```python
from build123d import *

# Parameters (mm, degrees)
EXTRUDE032_DEPTH           = 3
EXTRUDE033_DEPTH           = 3
CYLINDER057_R              = 4
CYLINDER057_DEPTH          = 12
CYLINDER055_R              = 4
CYLINDER055_DEPTH          = 12
CYLINDER053_R              = 1.85
CYLINDER053_DEPTH          = 12
CYLINDER054_R              = 1.85
CYLINDER054_DEPTH          = 12
CYLINDER056_R              = 4
CYLINDER056_DEPTH          = 12
CYLINDER052_R              = 1.85
CYLINDER052_DEPTH          = 12
EXTRUDE035_DEPTH           = 18
EXTRUDE035_PLACEMENT_ANGLE = 90
EXTRUDE034_DEPTH           = 18
EXTRUDE034_PLACEMENT_ANGLE = 90
BOX019_W                   = 75
BOX019_H                   = 150
BOX019_DEPTH               = 25
FILLET017_R                = 9.5
BOX018_W                   = 85
BOX018_H                   = 122
BOX018_DEPTH               = 12
FILLET016_R                = 3


with BuildPart() as batterybackattachpocket:
    # Sketch007 → Extrude032 (new body)
    with BuildSketch(Plane.XY):
        with BuildLine():
            ThreePointArc((-3, 0), (-2.12132, -2.12132), (0, -3))
            Line((0, -3), (0, -5))
            ThreePointArc((-5, 0), (-3.535534, -3.535534), (0, -5))
            Line((-5, 0), (-3, 0))
        make_face()
    extrude(amount=EXTRUDE032_DEPTH)


with BuildPart() as batterybackattachpocket_1:
    # Extrude032 placement: moved
    add(batterybackattachpocket.part.moved(Location((42.5, 45, -6))))


with BuildPart() as batterybackattachpocketleft:
    # Part__Mirroring004: instance of BatteryBackAttachPocket
    add(batterybackattachpocket_1.part.mirror(Plane(origin=(0, 0, 0), x_dir=(0, -1, 0), z_dir=(1, 0, 0))))


with BuildPart() as batterybackattachpocketright:
    # Sketch008 → Extrude033 (new body)
    with BuildSketch(Plane.XY):
        with BuildLine():
            ThreePointArc((-3, 0), (-2.12132, -2.12132), (0, -3))
            Line((0, -3), (0, -5))
            ThreePointArc((-5, 0), (-3.535534, -3.535534), (0, -5))
            Line((-5, 0), (-3, 0))
        make_face()
    extrude(amount=EXTRUDE033_DEPTH)


with BuildPart() as batterybackattachpocketright_1:
    # Extrude033 placement: moved
    add(batterybackattachpocketright.part.moved(Location((42.5, 45, -6))))


with BuildPart() as batterybackscrewcountersink3:
    # Cylinder057 → Cylinder057 (new body)
    with BuildSketch(Plane(origin=(34, -25, -1.5), x_dir=(-1, 0, 0), z_dir=(0, 0, -1))):
        Circle(CYLINDER057_R)
    extrude(amount=CYLINDER057_DEPTH)


with BuildPart() as batterybackscrewcountersink1:
    # Cylinder055 → Cylinder055 (new body)
    with BuildSketch(Plane(origin=(0, 41.5, -1.5), x_dir=(-1, 0, 0), z_dir=(0, 0, -1))):
        Circle(CYLINDER055_R)
    extrude(amount=CYLINDER055_DEPTH)


with BuildPart() as batterybackscrewhole2:
    # Cylinder053 → Cylinder053 (new body)
    with BuildSketch(Plane(origin=(-34, -25, 0), x_dir=(-1, 0, 0), z_dir=(0, 0, -1))):
        Circle(CYLINDER053_R)
    extrude(amount=CYLINDER053_DEPTH)


with BuildPart() as batterybackscrewhole3:
    # Cylinder054 → Cylinder054 (new body)
    with BuildSketch(Plane(origin=(34, -25, 0), x_dir=(-1, 0, 0), z_dir=(0, 0, -1))):
        Circle(CYLINDER054_R)
    extrude(amount=CYLINDER054_DEPTH)


with BuildPart() as batterybackscrewcountersink2:
    # Cylinder056 → Cylinder056 (new body)
    with BuildSketch(Plane(origin=(-34, -25, -1.5), x_dir=(-1, 0, 0), z_dir=(0, 0, -1))):
        Circle(CYLINDER056_R)
    extrude(amount=CYLINDER056_DEPTH)


with BuildPart() as batterymountingpockets:
    # Cylinder052 → Cylinder052 (new body)
    with BuildSketch(Plane(origin=(0, 41.5, 0), x_dir=(-1, 0, 0), z_dir=(0, 0, -1))):
        Circle(CYLINDER052_R)
    extrude(amount=CYLINDER052_DEPTH)

    # Fusion048: union BatteryBackScrewCountersink3, BatteryBackScrewCountersink1, BatteryBackScrewHole2, BatteryBackScrewHole3, BatteryBackScrewCountersink2
    add(batterybackscrewcountersink3.part)
    add(batterybackscrewcountersink1.part)
    add(batterybackscrewhole2.part)
    add(batterybackscrewhole3.part)
    add(batterybackscrewcountersink2.part)


with BuildPart() as batterybackstrappocketleft:
    # Sketch010 → Extrude035 (new body)
    with BuildSketch(Plane.XZ):
        with BuildLine():
            ThreePointArc((-3.5, 0), (-2.474874, -2.474874), (0, -3.5))
            Line((0, -3.5), (0, -5))
            ThreePointArc((-5, 0), (-3.535534, -3.535534), (0, -5))
            Line((-5, 0), (-3.5, 0))
        make_face()
    extrude(amount=-EXTRUDE035_DEPTH)


with BuildPart() as batterybackstrappocketleft_1:
    # Extrude035 placement: moved
    add(batterybackstrappocketleft.part.moved(Location((42.5, -2, -12))).rotate(Axis((42.5, -2, -12), (0, 1, 0)), EXTRUDE035_PLACEMENT_ANGLE))


with BuildPart() as batterybackstrappocket:
    # Sketch009 → Extrude034 (new body)
    with BuildSketch(Plane.XZ):
        with BuildLine():
            ThreePointArc((-3.5, 0), (-2.474874, -2.474874), (0, -3.5))
            Line((0, -3.5), (0, -5))
            ThreePointArc((-5, 0), (-3.535534, -3.535534), (0, -5))
            Line((-5, 0), (-3.5, 0))
        make_face()
    extrude(amount=-EXTRUDE034_DEPTH)


with BuildPart() as batterybackstrappocket_1:
    # Extrude034 placement: moved
    add(batterybackstrappocket.part.moved(Location((42.5, -2, -12))).rotate(Axis((42.5, -2, -12), (0, 1, 0)), EXTRUDE034_PLACEMENT_ANGLE))


with BuildPart() as batterybackstrappocketright:
    # Part__Mirroring005: instance of BatteryBackStrapPocket
    add(batterybackstrappocket_1.part.mirror(Plane(origin=(0, 0, 0), x_dir=(0, -1, 0), z_dir=(1, 0, 0))))


with BuildPart() as batterybackcombinedpockets:
    # Box019 → Box019 (new body)
    with BuildSketch(Plane(origin=(-37.5, -73, -29), x_dir=(1, 0, 0), z_dir=(0, 0, 1))):
        with Locations((37.5, 75)):
            Rectangle(BOX019_W, BOX019_H)
    extrude(amount=BOX019_DEPTH)

    # Fillet017
    fillet017_edges = [batterybackcombinedpockets.edges().sort_by_distance(p)[0] for p in [
        (-37.5, -73, -16.5),
        (-37.5, 2, -4),
        (-37.5, 77, -16.5),
        (-37.5, 2, -29),
        (37.5, -73, -16.5),
        (37.5, 2, -4),
        (37.5, 77, -16.5),
        (37.5, 2, -29),
        (0, -73, -29),
        (0, -73, -4),
        (0, 77, -29),
        (0, 77, -4),
    ]]
    fillet(fillet017_edges, radius=FILLET017_R)

    # Fusion049: union BatteryBackAttachPocketLeft, BatteryBackAttachPocketRight, BatteryMountingPockets, BatteryBackStrapPocketLeft, BatteryBackStrapPocketRight
    add(batterybackattachpocketleft.part)
    add(batterybackattachpocketright_1.part)
    add(batterymountingpockets.part)
    add(batterybackstrappocketleft_1.part)
    add(batterybackstrappocketright.part)


with BuildPart() as obj1:
    # Box018 → Box018 (new body)
    with BuildSketch(Plane(origin=(-42.5, -77, -12), x_dir=(1, 0, 0), z_dir=(0, 0, 1))):
        with Locations((42.5, 61)):
            Rectangle(BOX018_W, BOX018_H)
    extrude(amount=BOX018_DEPTH)

    # Fillet016
    fillet016_edges = [obj1.edges().sort_by_distance(p)[0] for p in [
        (-42.5, -77, -6),
        (-42.5, 45, -6),
        (-42.5, -16, -12),
        (42.5, -77, -6),
        (42.5, 45, -6),
        (42.5, -16, -12),
        (0, -77, -12),
        (0, 45, -12),
    ]]
    fillet(fillet016_edges, radius=FILLET016_R)

    # Cut013: cut BatteryBackCombinedPockets
    add(batterybackcombinedpockets.part, mode=Mode.SUBTRACT)


solid = obj1.part
```
The listing builds one solid part. Answer for the finished solid, in the listing's coordinates (mm). A direction names the side the tool comes from. Give positions to 0.01 mm unless a question says otherwise; leave off trailing zeros. Order: outer loops, then holes, each group sorted by start corner. A loop starts at its lowest first (then second) coordinate and runs counter-clockwise, first axis right, second up. Notation, with made-up numbers: (71.5, -27.75) - (116.5, -27.75) arc R14 cw to (116.5, -20.75) - close; hole circle Ø1 at (77, 56.5). An arc over 180 degrees is marked (long way). Use one line per item in the form item = value. Start each with the question number.
(1) A cutting plane is placed at A-A, the plane y = 12. Write down the section's boundary in (x, z).
(2) A cutting plane is placed at D-D, the plane y = 33.5. Write down the section's boundary in (x, z).
(3) A cutting plane is placed at B-B, the plane x = 0. Write down the section's boundary in (y, z), then the cut area to 3 significant figures.
(4) For faces 1 (the cylindrical face through (-37.815, -23.799, -5.51)), 2 (the cylindrical face through (-40.05, 6.87, -9.5)), 3 (the cylindrical face through (0.4, -69.7, -6.3)), determine the directions among +Z, -Z, +X, -X, +Y, -Y from which every point of the face is accessible in a straight line to the end or side of a thin tool.
(5) The mould has two halves that part along Y. Classify faces 4 (the flat face through (-1, -77, -5)), 5 (the flat face through (0, -8, -4)), 6 (the cylindrical face through (-41.64, 44.1, -4.44)), 7 (the flat face through (-36, -26, -1.5)): released by +Y, released by -Y, zero draft, split by the parting line, or undercut.
(6) Flat-ended cylindrical pins translate along their axes: pin 1 Ø1.5 at (x, y) = (-40, 42) entering from +Z; pin 2 Ø5 at (x, y) = (-34, -25) entering from -Z; pin 3 Ø1.5 at (x, y) = (8, -15.5) entering from -Z; pin 4 Ø2.5 at (x, z) = (41, -10.5) entering from +Y. Find the tip coordinate at first contact, or state that the pin passes through.
(7) A cutting plane is placed at C-C, the plane x = 17.5. Write down the section's boundary in (y, z).
(8) Consider line 1 (X direction, y = -25, z = -0.45); line 2 (Y direction, x = -34, z = -5.5); line 3 (Y direction, x = 0, z = -1.15). Determine where each line is inside the solid, lowest interval first. Write a range as from..to.
Ans:
q1.outline = (-42.5, -9) arc R3 ccw to (-39.5, -12) - (-39, -12) arc R3.5 ccw to (-42.5, -8.5) - close; (-42.5, -7) arc R5 cw to (-37.5, -12) - (-37.38, -12) arc R9.5 cw to (-28, -4) - (28, -4) arc R9.5 cw to (37.38, -12) - (37.5, -12) arc R5 cw to (42.5, -7) - (42.5, 0) - (-42.5, 0) - close; (39, -12) - (39.5, -12) arc R3 ccw to (42.5, -9) - (42.5, -8.5) arc R3.5 ccw to start
q2.outline = (-42.5, -9) arc R3 ccw to (-39.5, -12) - (-37.38, -12) arc R9.5 cw to (-28, -4) - (28, -4) arc R9.5 cw to (37.38, -12) - (39.5, -12) arc R3 ccw to (42.5, -9) - (42.5, 0) - (-42.5, 0) - close
q3.outline = (-77, -9) arc R3 ccw to (-74, -12) - (-72.88, -12) arc R9.5 cw to (-63.5, -4) - (37.5, -4) - (37.5, -1.5) - (39.65, -1.5) - (39.65, 0) - (-77, 0) - close; (43.35, -1.5) - (45, -1.5) - (45, 0) - (43.35, 0) - close
q3.area = 513 mm^2
q4.face_1 = -Z
q4.face_2 = none
q4.face_3 = -Z, +Y
q5.face_4 = released by -Y
q5.face_5 = zero draft
q5.face_6 = released by +Y
q5.face_7 = undercut
q6.pin_1 = 0
q6.pin_2 = -1.5
q6.pin_3 = -4
q6.pin_4 = 44.87
q7.outline = (-77, -9) arc R3 ccw to (-74, -12) - (-72.88, -12) arc R9.5 cw to (-63.5, -4) - (45, -4) - (45, 0) - (-77, 0) - close
q8.line_1 = -42.5..-35.85, -32.15..32.15, 35.85..42.5
q8.line_2 = -77..-29, -21..45
q8.line_3 = -77..39.65, 43.35..45
